For this review, take the finished solid that the model builds, in its own axes (mm). A direction names the side the tool comes from. Round coordinates to 2 decimals unless told otherwise and drop trailing zeros. Order: outer loops, then holes, each group sorted by start corner. A loop starts at its lowest first (then second) coordinate and runs counter-clockwise, first axis right, second up. Notation, with made-up numbers: (-27, 1.5) -> (-10, 1.5) arc R20 cw to (-10, 7.5) -> close; hole circle Ø7 at (84, -5.5). An arc over 180 degrees is marked (long way). Answer in a Markdown table with one row per item.
Autodesk Inventor part; units mm, degrees
ref_plane "YZ Plane" through (0, 0, 0) normal (1, 0, 0) x (0, 1, 0)
ref_plane "XZ Plane" through (0, 0, 0) normal (0, 1, 0) x (-1, 0, 0)
ref_plane "XY Plane" through (0, 0, 0) normal (0, 0, 1) x (1, 0, 0)
sketch "Esquisse1" plane through (0, 0, 0) normal (0, 1, 0) x (-1, 0, 0)
  line L0 (0, 0) -> (120, 0)
  line L1 (120, 180) -> (0, 180)
  line L2 (0, 180) -> (0, 0)
  arc A0 (120, 0) -> (120, 180) centre (120, 90) ccw
  circle A1 centre (120, 90) radius 60
  line L3 (120, 177) -> (3, 177)
  line L4 (3, 177) -> (3, 3)
  line L5 (3, 3) -> (120, 3)
  arc A2 (120, 3) -> (120, 177) centre (120, 90) ccw
  dimension "d2" = 120
  dimension "d3" = 120
  dimension "d4" = 180
  dimension "d5" = 3
extrude "Extrusion1" add sketch "Esquisse1" along normal blind 2 contours L2 L1 A0 L0 | A2 L5 L4 L3
sketch "Esquisse2" plane through (0, 2, 0) normal (0, 1, 0) x (1, 0, 0)
  arc A0 (-120, 0) -> (-120, -180) centre (-120, -90) ccw
  arc A1 (-120, 0) -> (-120, -180) centre (-120, -90) ccw
  line L0 (-120, -180) -> (0, -180)
  line L1 (-120, -180) -> (0, -180)
  line L2 (0, -180) -> (0, 0)
  line L3 (0, 0) -> (-120, 0)
  line L4 (0, 0) -> (-120, 0)
  arc A2 (-120, -3) -> (-120, -177) centre (-120, -90) ccw
  line L5 (-120, -3) -> (0, -3)
  line L6 (-3, -3) -> (-3, -177)
  line L7 (-3, -177) -> (-120, -177)
  arc A3 (-120, -3) -> (-120, -177) centre (-120, -90) ccw
  line L8 (-120, -3) -> (-3, -3)
  dimension "d8" = 3
  dimension "d9" = 90
  dimension "d10" = 3
extrude "Extrusion2" add sketch "Esquisse2" along normal blind 12
sketch "Esquisse3" plane through (0, 14, 0) normal (0, 1, 0) x (1, 0, 0)
  line L0 (-120, -180) -> (0, -180)
  line L1 (-7.3436, -180) -> (-19.3436, -180)
  line L2 (-19.3436, -180) -> (-19.3436, -192)
  line L3 (-19.3436, -192) -> (-7.3436, -192)
  line L4 (-7.3436, -192) -> (-7.3436, -180)
  circle A0 centre (-13.3436, -186) radius 2
  circle A1 centre (-120, -90) radius 60
  line L5 (-120, -90) -> (-228.3107, -90)
  line L6 (-19.3436, 0) -> (-19.3436, 12)
  line L7 (-19.3436, 12) -> (-7.3436, 12)
  line L8 (-7.3436, 12) -> (-7.3436, 0)
  circle A2 centre (-13.3436, 6) radius 2
  line L9 (-60, -180) -> (-60, 26.6941)
  line L10 (-112.6564, -180) -> (-100.6564, -180)
  line L11 (-100.6564, -180) -> (-100.6564, -192)
  line L12 (-100.6564, -192) -> (-112.6564, -192)
  line L13 (-112.6564, -192) -> (-112.6564, -180)
  circle A3 centre (-106.6564, -186) radius 2
  line L14 (-100.6564, 12) -> (-112.6564, 12)
  line L15 (-112.6564, 12) -> (-112.6564, 0)
  circle A4 centre (-106.6564, 6) radius 2
  line L16 (-100.6564, 12) -> (-100.6564, 0)
  line L17 (0, 0) -> (-120, 0)
  line L18 (-7.3436, 0) -> (-19.3436, 0)
  dimension "d13" = 12
  dimension "d14" = 12
  dimension "d15" = 4
extrude "Extrusion3" add sketch "Esquisse3" against normal blind 3 contours L17 L15 L14 L16 | L6 L7 L8 L17 | L0 L4 L3 L2 | L0 L11 L12 L13
properties part number "Socle"
Q1. Take a section at B-B, the plane y = 6.5. Write out the cut boundary in (x, z).
Answer key:
| item | result |
|---|---|
| outline | (-120, 0) -> (0, 0) -> (0, 180) -> (-120, 180) arc R90 ccw to start; hole (-120, 3) -> (-3, 3) -> (-3, 177) -> (-120, 177) arc R87 ccw to start |
Q2. The part is to be moulded in two halves that separate along Z. For faces 4 (the face through (-206.98, 7.92, 91.91)), 5 (the face through (-107, 11, -9)), 6 (the face through (-209.98, 6.9, 91.98)), say which applies: +Z half, -Z half, draft (parallel to the pull), parting line (faces both ways), or undercut.
Answer key:
| item | result |
|---|---|
| face 4 | undercut |
| face 5 | draft |
| face 6 | parting line |
Q3. Take a section at A-A, the plane z = 90. Write out the cut boundary in (x, y), then the cut area to 3 significant figures.
Answer key:
| item | result |
|---|---|
| outline | (-210, 0) -> (-180, 0) -> (-180, 2) -> (-207, 2) -> (-207, 14) -> (-210, 14) -> close; (-60, 0) -> (0, 0) -> (0, 14) -> (-3, 14) -> (-3, 2) -> (-60, 2) -> close |
| area | 252 mm^2 |
Q4. Clearance check with flat-ended pins moving along their axes: pin 1 Ø5 at (y, z) = (3, 167.5) entering from -X; pin 2 Ø0.9 at (y, z) = (12.5, 188.5) entering from -X; pin 3 Ø3 at (x, y) = (-151.5, 5.5) entering from +Z. State where each tip first meets the part, or that it passes through.
Answer key:
| item | result |
|---|---|
| pin 1 | stops at x = -169.75 |
| pin 2 | stops at x = -112.66 |
| pin 3 | stops at z = 174.85 |
Q5. To check wall thickness, follow probe 1 along X at (y, z) = (12.2, 186); probe 2 along Z at (x, y) = (-19.5, 6.5); probe 3 along Y at (x, z) = (-40.5, 4). State the ranges of each line that lie inside material, in increasing order.
Answer key:
| item | result |
|---|---|
| probe 1 | x = -112.66 to -108.66, -104.66 to -100.66, -19.34 to -15.34, -11.34 to -7.34 |
| probe 2 | z = 0 to 3, 177 to 180 |
| probe 3 | y = 0 to 2 |
Q6. Take a section at D-D, the plane x = -82. Write out the cut boundary in (y, z), then the cut area to 3 significant figures.
Answer key:
| item | result |
|---|---|
| outline | (0, 0) -> (14, 0) -> (14, 3) -> (2, 3) -> (2, 43.57) -> (0, 43.57) -> close; (0, 136.43) -> (2, 136.43) -> (2, 177) -> (14, 177) -> (14, 180) -> (0, 180) -> close |
| area | 246 mm^2 |
Q7. Take a section at C-C, the plane x = -54.5. Write out the cut boundary in (y, z), then the cut area to 3 significant figures.
Answer key:
| item | result |
|---|---|
| outline | (0, 0) -> (14, 0) -> (14, 3) -> (2, 3) -> (2, 177) -> (14, 177) -> (14, 180) -> (0, 180) -> close |
| area | 432 mm^2 |
Q8. Tool access review of faces 1 (the face through (-107, 11, 183)), 2 (the face through (-13, 11, -9)), 3 (the face through (-58, 2, 91)): name each direction out of +Z, -Z, +X, -X, +Y, -Y from which nothing blocks a thin tool from reaching the whole face with its end or side.
Answer key:
| item | result |
|---|---|
| face 1 | +Z, +X, -X, -Y |
| face 2 | -Z, +X, -X, -Y |
| face 3 | +Y |
